from build123d import *

# Parameters (mm, degrees)
SKETCH1_W                                  = 700
SKETCH1_H                                  = 700
SKETCH1_W_2                                = 500
SKETCH1_H_2                                = 500
BOSS_EXTRUDE2_DEPTH                        = 50
BOSS_EXTRUDE2_DRAFT                        = 45
SKETCH6_W                                  = 700
SKETCH6_H                                  = 700
SKETCH6_W_2                                = 600
SKETCH6_H_2                                = 600
CUT_EXTRUDE1_DEPTH                         = 50
CUT_EXTRUDE2_DEPTH                         = 25
SKETCH8_R                                  = 2.5
BOSS_EXTRUDE3_DEPTH                        = 10
MIRROR1_AT_THE_SECOND_PLANE_COPY_1_SKETC_R = 2.5
MIRROR1_AT_THE_SECOND_PLANE_COPY_1_DEPTH   = 10
MIRROR2_COPY_1_SKETCH_R                    = 2.5
MIRROR2_COPY_1_DEPTH                       = 10
MIRROR2_COPY_2_SKETCH_R                    = 2.5
MIRROR2_COPY_2_DEPTH                       = 10
MIRROR2_COPY_3_SKETCH_R                    = 2.5
MIRROR2_COPY_3_DEPTH                       = 10
SKETCH9_W                                  = 25
SKETCH9_H                                  = 15
BOSS_EXTRUDE4_DEPTH                        = 30
SKETCH11_R                                 = 12.5
BOSS_EXTRUDE5_DEPTH                        = 50
FILLET1_R                                  = 12.5
FILLET1_OF_MIRROR3_R                       = 12.5
MIRROR4_START                              = -25
MIRROR4_OUTLINE_R                          = 12.5
MIRROR4_DEPTH                              = 50
MIRROR4_2_DEPTH                            = 15
MIRROR4_START_2                            = 10
MIRROR4_3_DEPTH                            = 15


# Read off the part's stored shape, not the designer's step: Mirror4
with BuildPart() as part:
    # Sketch1 → Boss-Extrude2 (with draft: the straight prism first)
    with BuildSketch(Plane(origin=(0, 0, 0), x_dir=(1, 0, 0), z_dir=(0, 1, 0))):
        Rectangle(SKETCH1_W, SKETCH1_H)
        Rectangle(SKETCH1_W_2, SKETCH1_H_2, mode=Mode.SUBTRACT)
    extrude(amount=BOSS_EXTRUDE2_DEPTH)
    # Boss-Extrude2: the draft: its side faces are tilted about the plane it starts from
    boss_extrude2_sides = [part.faces().sort_by_distance(p)[0] for p in [
        (-350, 25, 0),
        (0, 25, 350),
        (350, 25, 0),
        (0, 25, -350),
        (250, 25, 0),
        (0, 25, 250),
        (-250, 25, 0),
        (0, 25, -250),
    ]]
    draft(boss_extrude2_sides, Plane(origin=(0, 0, 0), x_dir=(1, 0, 0), z_dir=(0, 1, 0)), BOSS_EXTRUDE2_DRAFT)

    # Sketch6 → Cut-Extrude1 (cut)
    with BuildSketch(Plane(origin=(0, 50, 0), x_dir=(1, 0, 0), z_dir=(0, 1, 0))):
        Rectangle(SKETCH6_W, SKETCH6_H)
        Rectangle(SKETCH6_W_2, SKETCH6_H_2, mode=Mode.SUBTRACT)
    extrude(amount=-CUT_EXTRUDE1_DEPTH, mode=Mode.SUBTRACT)

    # Sketch7 → Cut-Extrude2 (cut)
    with BuildSketch(Plane.XZ):
        Polygon((-275, 250), (-250, 250), (-250, 275), (250, 275), (250, 250), (275, 250), (275, -250), (250, -250), (250, -275), (-250, -275), (-250, -250), (-275, -250), align=None)
    extrude(amount=-CUT_EXTRUDE2_DEPTH, mode=Mode.SUBTRACT)

    # Sketch8 → Boss-Extrude3 (add)
    with BuildSketch(Plane.XY.offset(-250)):
        with Locations(Location((-268.75, 6.25, 0), (0, 0, 180))):
            Circle(SKETCH8_R)
    boss_extrude3 = extrude(amount=BOSS_EXTRUDE3_DEPTH)

    # Mirror1: Boss-Extrude3 across plane
    add(boss_extrude3.mirror(Plane(origin=(0, 0, 0), x_dir=(0, 0, 1), z_dir=(1, 0, 0))))

    # Mirror1 at the second plane: Boss-Extrude3 across plane
    add(boss_extrude3.mirror(Plane.XY))

    # Mirror1 at the second plane copy 1 sketc → Mirror1 at the second plane copy 1 (add)
    with BuildSketch(Plane(origin=(0, 0, 250), x_dir=(-1, 0, 0), z_dir=(0, 0, -1))):
        with Locations(Location((-268.75, 6.25, 0), (0, 0, 180))):
            Circle(MIRROR1_AT_THE_SECOND_PLANE_COPY_1_SKETC_R)
    extrude(amount=MIRROR1_AT_THE_SECOND_PLANE_COPY_1_DEPTH)

    # Mirror2: Boss-Extrude3 across plane
    add(boss_extrude3.mirror(Plane(origin=(0, 0, 0), x_dir=(0.7071067811865477, 0, 0.7071067811865474), z_dir=(-0.7071067811865474, 0, 0.7071067811865477))))

    # Mirror2 copy 1 sketch → Mirror2 copy 1 (add)
    with BuildSketch(Plane(origin=(-250, 0, 0), x_dir=(0, 0, -1), z_dir=(1, 0, 0))):
        with Locations(Location((-268.75, 6.25, 0), (0, 0, 180))):
            Circle(MIRROR2_COPY_1_SKETCH_R)
    extrude(amount=MIRROR2_COPY_1_DEPTH)

    # Mirror2 copy 2 sketch → Mirror2 copy 2 (add)
    with BuildSketch(Plane.ZY.offset(-250)):
        with Locations(Location((-268.75, 6.25, 0), (0, 0, 180))):
            Circle(MIRROR2_COPY_2_SKETCH_R)
    extrude(amount=MIRROR2_COPY_2_DEPTH)

    # Mirror2 copy 3 sketch → Mirror2 copy 3 (add)
    with BuildSketch(Plane(origin=(250, 0, 0), x_dir=(0, 0, -1), z_dir=(-1, 0, 0))):
        with Locations((-268.75, -6.25)):
            Circle(MIRROR2_COPY_3_SKETCH_R)
    extrude(amount=MIRROR2_COPY_3_DEPTH)

    # Sketch9 → Boss-Extrude4 (add)
    with BuildSketch(Plane.XZ):
        with Locations((-287.5, 17.5)):
            Rectangle(SKETCH9_W, SKETCH9_H)
        with Locations((-287.5, -17.5)):
            Rectangle(SKETCH9_W, SKETCH9_H)
    boss_extrude4 = extrude(amount=BOSS_EXTRUDE4_DEPTH)

    # Sketch11 → Boss-Extrude5 (add)
    with BuildSketch(Plane(origin=(0, 0, -25), x_dir=(-1, 0, 0), z_dir=(0, 0, -1))):
        with Locations((287.5, -17.5)):
            Circle(SKETCH11_R)
    boss_extrude5 = extrude(amount=-BOSS_EXTRUDE5_DEPTH)

    # Fillet1
    fillet1_edges = [part.edges().sort_by_distance(p)[0] for p in [
        (-275, -30, -17.5),
        (-275, -30, 17.5),
        (-300, -30, 17.5),
        (-300, -30, -17.5),
    ]]
    fillet(fillet1_edges, radius=FILLET1_R - 0.0001)  # a hair under: the kernel refuses the full size

    # Mirror3: Boss-Extrude4, Boss-Extrude5 across plane
    add(boss_extrude4.mirror(Plane(origin=(0, 0, 0), x_dir=(0, 0, 1), z_dir=(1, 0, 0))))
    add(boss_extrude5.mirror(Plane(origin=(0, 0, 0), x_dir=(0, 0, 1), z_dir=(1, 0, 0))))

    # Fillet1 of Mirror3
    fillet1_of_mirror3_edges = [part.edges().sort_by_distance(p)[0] for p in [
        (275, -30, -17.5),
        (275, -30, 17.5),
        (300, -30, 17.5),
        (300, -30, -17.5),
    ]]
    fillet(fillet1_of_mirror3_edges, radius=FILLET1_OF_MIRROR3_R - 0.0001)  # a hair under: the kernel refuses the full size



with BuildPart() as body_2:
    # Mirror4 outline → Mirror4 (new body)
    with BuildSketch(Plane.YZ.offset(MIRROR4_START)):
        with Locations((-17.5, 287.5)):
            Circle(MIRROR4_OUTLINE_R)
        with Locations((-17.5, -287.5)):
            Circle(MIRROR4_OUTLINE_R)
    extrude(amount=MIRROR4_DEPTH)


with BuildPart() as part_1:
    add(part.part)

    add(body_2.part)  # Mirror4 2 merges body 2
    # Mirror4 2 outline → Mirror4 2 (add)
    with BuildSketch(Plane.YZ.offset(MIRROR4_START)):
        with BuildLine():
            ThreePointArc((-17.5, 300), (-5, 287.5), (-17.5, 275))
            Line((-17.5, 275), (0, 275))
            Line((0, 275), (0, 300))
            Line((0, 300), (-17.5, 300))
        make_face()
        with BuildLine():
            ThreePointArc((-17.5, -275), (-5, -287.5), (-17.5, -300))
            Line((-17.5, -300), (0, -300))
            Line((0, -300), (0, -275))
            Line((0, -275), (-17.5, -275))
        make_face()
    extrude(amount=MIRROR4_2_DEPTH)

    # Mirror4 3 outline → Mirror4 3 (add)
    with BuildSketch(Plane.YZ.offset(MIRROR4_START_2)):
        with BuildLine():
            ThreePointArc((-17.5, 300), (-5, 287.5), (-17.5, 275))
            Line((-17.5, 275), (0, 275))
            Line((0, 275), (0, 300))
            Line((0, 300), (-17.5, 300))
        make_face()
        with BuildLine():
            ThreePointArc((-17.5, -275), (-5, -287.5), (-17.5, -300))
            Line((-17.5, -300), (0, -300))
            Line((0, -300), (0, -275))
            Line((0, -275), (-17.5, -275))
        make_face()
    extrude(amount=MIRROR4_3_DEPTH)


solid = part_1.part
Verification items for the finished model (mm, model axes). A direction names the side the tool comes from. Round coordinates to 2 decimals unless told otherwise and drop trailing zeros. Order: outer loops, then holes, each group sorted by start corner. A loop starts at its lowest first (then second) coordinate and runs counter-clockwise, first axis right, second up.
1. Section check A-A on z = 102.5. Record the cut outline in (x, y).
Final values:
outline: (-300, 0) - (-275, 0) - (-275, 25) - (-300, 50) - close; (275, 0) - (300, 0) - (300, 50) - (275, 25) - close
2. Thickness scan on L1, parallel to X at y = 15, z = 233; L2, parallel to Z at x = 178, y = 30. Record the ranges inside material, lowest first.
Final values:
L1: x = -300 to -275, 275 to 300
L2: z = -300 to -280, 280 to 300
3. Go/stop test with flat-tipped pins: P1, Ø14, axis at x = 282.5, y = -24.5, coming from the +Z side; P2, Ø5, axis at y = -10, z = 293, coming from the +X side; P3, Ø14, axis at x = -290, y = -8.5, coming from the -Z side. Record where each tip stops, or that it passes through.
Final values:
P1: stops at z = 25
P2: stops at x = 25
P3: stops at z = -25
4. Release check for a two-part mould opening along Y. For faces 5 (the flat face through (-4, 24, -300)), 6 (the flat face through (286, 36, 4)), 7 (the cylindrical face through (-0.35, -29.988, 288.05)) record: +Y half, -Y half, draft (parallel to the pull), parting line (faces both ways), or undercut.
Final values:
face 5: draft
face 6: +Y half
face 7: undercut
5. Section check B-B on x = 66. Record the cut outline in (y, z).
Final values:
outline: (0, -300) - (50, -300) - (25, -275) - (0, -275) - close; (0, 275) - (25, 275) - (50, 300) - (0, 300) - close
6. Section check C-C on y = 36. Record the cut outline in (x, z), then the cut area to 3 significant figures.
Final values:
outline: (-300, -300) - (300, -300) - (300, 300) - (-300, 300) - close; hole (-286, -286) - (286, -286) - (286, 286) - (-286, 286) - close
area: 32,800 mm2
7. Access from +Z, -Z, +X, -X, +Y, -Y to the whole of each face (thin tool, end or side, straight path). Record for faces 1 (the flat face through (-288, -15, 25)), 2 (the flat face through (254, 0, 264)), 3 (the flat face through (-286, 36, 4)), 4 (the flat face through (288, -15, -25)).
Final values:
face 1: +Z, +X, -X, -Y
face 2: +Z, +X, -Y
face 3: +Y
face 4: -Z, +X, -X, -Y
